Geometry: final body of the model. Coordinates: model frame, mm. Round coordinates to 2 decimals unless told otherwise and drop trailing zeros. Write each loop counter-clockwise with the first axis right and the second up, starting at its lowest first coordinate (ties: lowest second). Pieces come first, ordered by that corner, then holes.
Autodesk Inventor part; units mm, degrees
ref_plane "YZ Plane" through (0, 0, 0) normal (1, 0, 0) x (0, 1, 0)
ref_plane "XZ Plane" through (0, 0, 0) normal (0, 1, 0) x (-1, 0, 0)
ref_plane "XY Plane" through (0, 0, 0) normal (0, 0, 1) x (1, 0, 0)
sketch "Esboço1" plane through (0, 0, 0) normal (0, 1, 0) x (-1, 0, 0)
  line L0 (0, 0) -> (19.8493, 0)
  line L1 (19.8493, 0) -> (19.8493, -85)
  line L2 (19.8493, -85) -> (0, -85)
  line L3 (0, -85) -> (0, 0)
  line L4 (20, -22) -> (20, -63)
  line L5 (0, -63) -> (0, -22)
  circle A0 centre (14.8493, -75) radius 1.5
  circle A1 centre (5, -75) radius 1.5
  circle A2 centre (14.8493, -10) radius 1.5
  circle A3 centre (5, -10) radius 1.5
  dimension "d15" = 3
  dimension "d16" = 3
  dimension "d17" = 3
  dimension "d18" = 3
  dimension "d19" = 10
  dimension "d20" = 5
  dimension "d21" = 5
  dimension "d22" = 10
  dimension "d23" = 5
  dimension "d24" = 5
  dimension "d25" = 10
  dimension "d26" = 10
extrude "Extrusão3" add sketch "Esboço1" along normal blind 4
properties part number "suporte estruzor 2"
1) Section A-A on z = -75. Output: boundary loops of the cut face in (x, y).
2) Draft query along X for faces 1 (the cylindrical face through (-5.806, 1.972, -76.265)), 2 (the flat face through (0, 2, -43)), 3 (the cylindrical face through (-13.35, 1.97, -10.07)), 4 (the flat face through (-19.849, 2, -42)). Return one class per face: pulls with the +X half, pulls with the -X half, needs draft (parallel to the pull), parting line crosses it, or undercut.
3) First-contact query: P1, Ø2.5, axis at x = -14.85, z = -10, coming from the -Y side. Flat tip, straight axial feed; report the tip coordinate or a pass-through.
4) Section B-B on x = -5. Output: boundary loops of the cut face in (y, z).
5) Line query: probe 1 along X at (y, z) = (1.4, -75); probe 2 along Z at (x, y) = (-5, 3.15); probe 3 along Z at (x, y) = (-14, 2.4). Output: solid intervals per line, ascending.
6) Section C-C on y = 1.2. Output: boundary loops of the cut face in (x, z), plus the area to 3 significant figures.
Filled in:
1. outline: (-19.85, 0) - (-16.35, 0) - (-16.35, 4) - (-19.85, 4) - close; (-13.35, 0) - (-6.5, 0) - (-6.5, 4) - (-13.35, 4) - close; (-3.5, 0) - (0, 0) - (0, 4) - (-3.5, 4) - close
2. face 1: undercut
2. face 2: pulls with the +X half
2. face 3: undercut
2. face 4: pulls with the -X half
3. P1: passes through
4. outline: (0, -85) - (4, -85) - (4, -76.5) - (0, -76.5) - close; (0, -73.5) - (4, -73.5) - (4, -11.5) - (0, -11.5) - close; (0, -8.5) - (4, -8.5) - (4, 0) - (0, 0) - close
5. probe 1: x = -19.85 to -16.35, -13.35 to -6.5, -3.5 to 0
5. probe 2: z = -85 to -76.5, -73.5 to -11.5, -8.5 to 0
5. probe 3: z = -85 to -76.24, -73.76 to -11.24, -8.76 to 0
6. outline: (-19.85, -85) - (0, -85) - (0, 0) - (-19.85, 0) - close; hole circle Ø3 at (-14.85, -75); hole circle Ø3 at (-14.85, -10); hole circle Ø3 at (-5, -75); hole circle Ø3 at (-5, -10)
6. area: 1,660 mm2
